Input: dimensioned drawing with shaded views. Units: mm. Origin: part minimum x, y, z. Give positions to 0.01 mm unless a question says otherwise; leave off trailing zeros. Write each loop counter-clockwise with the first axis right and the second up, starting at its lowest first coordinate (ties: lowest second). Pieces come first, ordered by that corner, then holes. Notation, with made-up numbers: M -1,73 L 52,73 A26 cw 52,108 Z; hole C 28,-18.5 d7. An arc over 180 degrees is marked long. Answer as a JSON object with one key per item and string values.
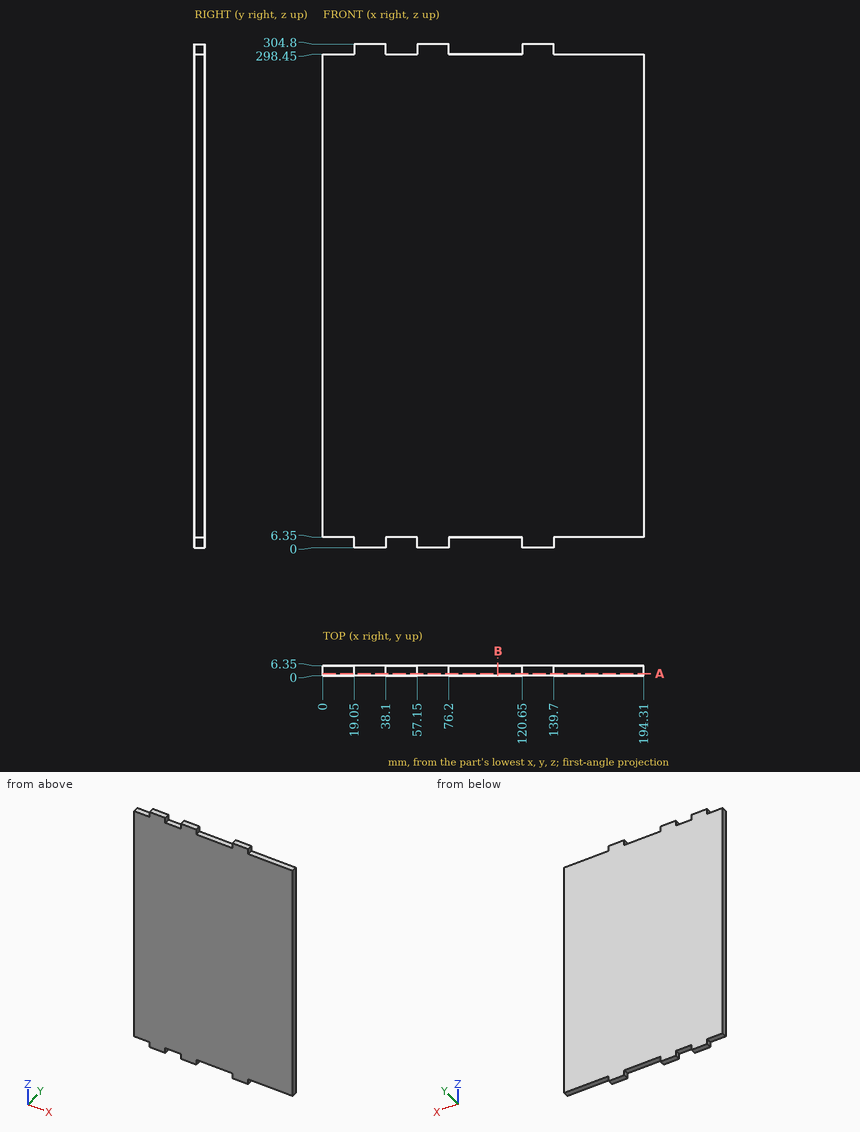
1) Cut plane B-B on x = 106. Return loops of the section in (y, z), and give its area (3 significant figures).
Geometry check:
{"outline": "M 0,6.35 L 6.35,6.35 L 6.35,298.45 L 0,298.45 Z", "area": "1,850 mm2"}
2) Contact query for flat-ended pins moving along their axis: P1, Ø1, axis at x = 95, y = 5.5, coming from the -Z side; P2, Ø2, axis at x = 171.5, y = 3, coming from the +Z side; P3, Ø10, axis at x = 127, z = 101.5, coming from the -Y side; P4, Ø3, axis at y = 2.5, z = 303, coming from the +X side. Output: stop coordinate, or through.
Geometry check:
{"P1": "stops at z = 6.35", "P2": "stops at z = 298.45", "P3": "stops at y = 0", "P4": "stops at x = 139.7"}
3) Line query: line 1 (Z direction, x = 77.5, y = 3.75). Output: solid intervals per line, ascending. Write a range as from..to.
Geometry check:
{"line 1": "z = 6.35..298.45"}
4) Cut plane A-A on y = 1.5. Return loops of the section in (x, z).
Geometry check:
{"outline": "M 0,6.35 L 19.05,6.35 L 19.05,0 L 38.1,0 L 38.1,6.35 L 57.15,6.35 L 57.15,0 L 76.2,0 L 76.2,6.35 L 120.65,6.35 L 120.65,0 L 139.7,0 L 139.7,6.35 L 194.31,6.35 L 194.31,298.45 L 139.7,298.45 L 139.7,304.8 L 120.65,304.8 L 120.65,298.45 L 76.2,298.45 L 76.2,304.8 L 57.15,304.8 L 57.15,298.45 L 38.1,298.45 L 38.1,304.8 L 19.05,304.8 L 19.05,298.45 L 0,298.45 Z"}
